Design review of the part built by this model. Coordinates are the model's own, in mm. Face numbers are marked on the shaded views. Coordinates: 2 decimals unless noted, no trailing zeros. Write each loop counter-clockwise with the first axis right and the second up, starting at its lowest first coordinate (ties: lowest second). Pieces come first, ordered by that corner, then holes. Notation, with made-up numbers: (30, -32.75) - (59, -32.75) arc R15 ccw to (59, -16.75) - close; hole circle Ø4 at (63.5, 37). An arc over 180 degrees is marked (long way). Answer as CSV lines item,"result". Start each with the question number.
Q1. Mouldability with a two-part tool opening along Z and no side actions: class the marked faces 1, 2 and 3 as pulls with the +Z half, pulls with the -Z half, needs draft (parallel to the pull), parting line crosses it, or undercut.
Q2. We need section B-B (x = 14). Write out the cut boundary in (y, z), plus the area to 3 significant figures.
Q3. Clearance check with a flat-ended pin moving along its axis: pin 1 (6.5 mm diameter, centred on x = 0, z = 0, fed in from -Y). State where the tip first meets the part, or that it passes through.
Q4. We need section D-D (x = 0). Write out the cut boundary in (y, z).
Q5. We need section A-A (z = 0). Write out the cut boundary in (x, y), plus the area to 3 significant figures.
Q6. We need section C-C (z = -6). Write out the cut boundary in (x, y).
Q7. For line 1 along X through (y, z) = (1.65, -7.25); line 2 along Y through (x, z) = (14, -1); line 3 along X through (y, z) = (3.8, -3), list the stretches that pass through material, from the lowest coordinate up. Write a range as [from, to].
Autodesk Inventor part; units mm, degrees
ref_plane "YZ Plane" through (0, 0, 0) normal (1, 0, 0) x (0, 1, 0)
ref_plane "XZ Plane" through (0, 0, 0) normal (0, 1, 0) x (-1, 0, 0)
ref_plane "XY Plane" through (0, 0, 0) normal (0, 0, 1) x (1, 0, 0)
sketch "Boceto1" plane through (0, 0, 0) normal (0, 1, 0) x (-1, 0, 0)
  line L0 (-37.5, 12.5) -> (37.5, 12.5)
  line L1 (37.5, 12.5) -> (37.5, -12.5)
  line L2 (37.5, -12.5) -> (-37.5, -12.5)
  line L3 (-37.5, -12.5) -> (-37.5, 12.5)
  line L4 (-37.5, 12.5) -> (37.5, -12.5) construction
  line L5 (37.5, 12.5) -> (-37.5, -12.5) construction
  point P0 (0, 0)
  dimension "d4" = 25
  dimension "d5" = 75
extrude "Extrusión1" add sketch "Boceto1" along normal blind 5
sketch "Boceto2" plane through (-37.5, 0, 12.5) normal (0, 0, 1) x (1, 0, 0)
  line L0 (75, 0) -> (0, 0)
  line L1 (75, 0) -> (75, 5)
  line L2 (0, 5) -> (75, 5)
  line L3 (0, 0) -> (0, 5)
  line L4 (37.5, 0) -> (37.5, 5)
  point P0 (23.5, 2.5)
  point P1 (16, 2.5)
  point P2 (51.5, 2.5)
  point P3 (59, 2.5)
  dimension "d12" = 14
  dimension "d13" = 21.5
hole "Agujero1" at (-14, 2.5, 12.5) at (14, 2.5, 12.5) direction (0, 0, -1) diameter 3 end through all
hole "Agujero2" at (-21.5, 2.5, 12.5) at (21.5, 2.5, 12.5) direction (0, 0, -1) diameter 2 depth 20 tip angle 118
sketch "Boceto3" plane through (0, 5, 0) normal (0, 1, 0) x (1, 0, 0)
  circle A0 centre (-21.5, 0) radius 5
  line L0 (0, -9.1996) -> (0, 9.6209)
  circle A1 centre (21.5, 0) radius 5
  circle A2 centre (0, 0) radius 4
  dimension "d28" = 21.5
  dimension "d29" = 0
  dimension "d30" = 10
  dimension "d31" = 0
  dimension "d34" = 8
  dimension "d35" = 0
  dimension "d36" = 0
extrude "Extrusión2" cut sketch "Boceto3" against normal through all
equation "\"d4\" = 25 * scale"
equation "\"d5\" = 75 * scale"
equation "\"d2\" = 5 * scale"
equation "\"d30\" = 10 * scale"
equation "\"d34\" = 8 * scale"
equation "\"scale\" = 1"
properties part number "Placa2"
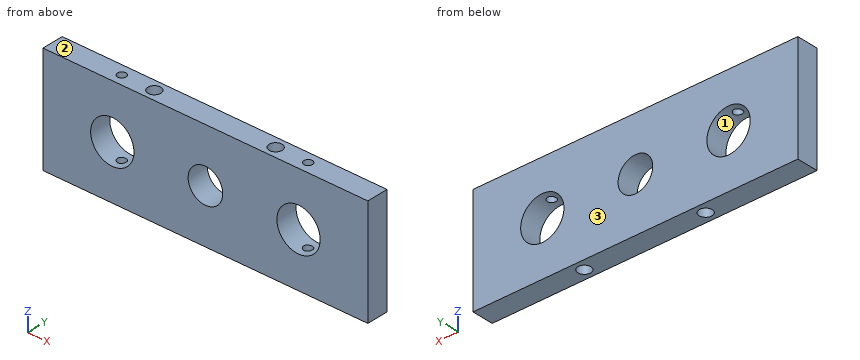
Results list:
1,face 1,"undercut"
1,face 2,"pulls with the +Z half"
1,face 3,"needs draft"
2,outline,"(0, -12.5) - (1, -12.5) - (1, 12.5) - (0, 12.5) - close; (4, -12.5) - (5, -12.5) - (5, 12.5) - (4, 12.5) - close"
2,area,"50.0 mm2"
3,pin 1,"passes through"
4,outline,"(0, -12.5) - (5, -12.5) - (5, -4) - (0, -4) - close; (0, 4) - (5, 4) - (5, 12.5) - (0, 12.5) - close"
5,outline,"(-37.5, 0) - (-26.5, 0) - (-26.5, 5) - (-37.5, 5) - close; (-16.5, 0) - (-4, 0) - (-4, 5) - (-16.5, 5) - close; (4, 0) - (16.5, 0) - (16.5, 5) - (4, 5) - close; (26.5, 0) - (37.5, 0) - (37.5, 5) - (26.5, 5) - close; hole circle Ø3 at (-14, 2.5); hole circle Ø3 at (14, 2.5)"
5,area,"221 mm2"
6,outline,"(-37.5, 0) - (37.5, 0) - (37.5, 5) - (-37.5, 5) - close; hole circle Ø2 at (-21.5, 2.5); hole circle Ø3 at (-14, 2.5); hole circle Ø3 at (14, 2.5); hole circle Ø2 at (21.5, 2.5)"
7,line 1,"x = [-37.5, -22.03], [-20.97, -15.24], [-12.76, 12.76], [15.24, 20.97], [22.03, 37.5]"
7,line 2,"y = [0, 1], [4, 5]"
7,line 3,"x = [-37.5, -25.5], [-17.5, -14.75], [-13.25, -2.65], [2.65, 13.25], [14.75, 17.5], [25.5, 37.5]"
